The model under review builds one solid part; all positions refer to its coordinate system, in mm. A direction names the side the tool comes from. Give positions to 0.01 mm unless a question says otherwise; leave off trailing zeros. Loops run counter-clockwise (first coordinate to the right, second up) from the corner with the lowest first, then second, coordinate; pieces in that order, holes last. Notation, with made-up numbers: (73.5, -18.75) - (91.5, -18.75) arc R15 cw to (91.5, -0.75) - close; hole circle Ø6 at (32.5, 45). An arc over 180 degrees is marked (long way). Answer as a JSON object with one key per item and string values.
from build123d import *

# Parameters (mm, degrees)
SKETCH1_W           = 88
SKETCH1_H           = 18
BOSS_EXTRUDE1_DEPTH = 3.8
SKETCH2_W           = 18.8
SKETCH2_H           = 3.8
BOSS_EXTRUDE2_DEPTH = 3.8
SKETCH3_W           = 10
SKETCH3_H           = 3.8
BOSS_EXTRUDE3_DEPTH = 3.8
LPATTERN1_COUNT     = 3
LPATTERN1_PITCH     = 20
LPATTERN1_COL_COUNT = 3
LPATTERN1_COL_PITCH = 20
SKETCH4_W           = 1
SKETCH4_H           = 3.8
CUT_EXTRUDE1_DEPTH  = 92.709759568
SKETCH5_W           = 88
SKETCH5_H           = 3
BOSS_EXTRUDE4_DEPTH = 3.8
SKETCH6_W           = 5
SKETCH6_H           = 3.8
BOSS_EXTRUDE5_DEPTH = 3.8
SKETCH7_W           = 10
SKETCH7_H           = 7.6
BOSS_EXTRUDE6_DEPTH = 3.8
LPATTERN2_COUNT     = 3
LPATTERN2_PITCH     = 20
SKETCH9_W           = 9
SKETCH9_H           = 3.8
CUT_EXTRUDE2_DEPTH  = 92.506721065
SKETCH10_W          = 3.8
SKETCH10_H          = 5
SKETCH10_H_2        = 8
BOSS_EXTRUDE8_DEPTH = 3.8
SKETCH11_W          = 10
SKETCH11_H          = 3
CUT_EXTRUDE3_DEPTH  = 96.166800934


with BuildPart() as part:
    # Sketch1 → Boss-Extrude1 (new body)
    with BuildSketch(Plane(origin=(0, 0, 0), x_dir=(1, 0, 0), z_dir=(0, 1, 0))):
        with Locations((44, -9)):
            Rectangle(SKETCH1_W, SKETCH1_H)
    extrude(amount=BOSS_EXTRUDE1_DEPTH)

    # Sketch2 → Boss-Extrude2 (add, through all)
    with BuildSketch(Plane.XZ):
        with Locations((9.4, -1.9)):
            Rectangle(SKETCH2_W, SKETCH2_H)
    extrude(amount=-BOSS_EXTRUDE2_DEPTH)

    # Sketch3 → Boss-Extrude3 (add, through all)
    with BuildSketch(Plane.XZ):
        with Locations((44, 19.9)):
            Rectangle(SKETCH3_W, SKETCH3_H)
    boss_extrude3 = extrude(amount=-BOSS_EXTRUDE3_DEPTH)

    # LPattern1: Boss-Extrude3 ×3
    with Locations(*[(i * LPATTERN1_PITCH, 0, 0) for i in range(1, LPATTERN1_COUNT)]):
        add(boss_extrude3)

    # LPattern1 col: Boss-Extrude3 ×3
    with Locations(*[(-i * LPATTERN1_COL_PITCH, 0, 0) for i in range(1, LPATTERN1_COL_COUNT)]):
        add(boss_extrude3)

    # Sketch4 → Cut-Extrude1 (cut, through all)
    with BuildSketch(Plane(origin=(0, 0, 0), x_dir=(-1, 0, 0), z_dir=(0, -1, 0))):
        with Locations((0.5, -19.9)):
            Rectangle(SKETCH4_W, SKETCH4_H)
        with Locations((-88.5, -19.9)):
            Rectangle(SKETCH4_W, SKETCH4_H)
    extrude(amount=-CUT_EXTRUDE1_DEPTH, mode=Mode.SUBTRACT)

    # Sketch5 → Boss-Extrude4 (add, through all)
    with BuildSketch(Plane(origin=(0, 0, 0), x_dir=(-1, 0, 0), z_dir=(0, -1, 0))):
        with Locations((-44, -23.3)):
            Rectangle(SKETCH5_W, SKETCH5_H)
    extrude(amount=-BOSS_EXTRUDE4_DEPTH)

    # Sketch6 → Boss-Extrude5 (add, through all)
    with BuildSketch(Plane(origin=(0, 0, 0), x_dir=(-1, 0, 0), z_dir=(0, -1, 0))):
        with Locations((-2.5, 5.7)):
            Rectangle(SKETCH6_W, SKETCH6_H)
        with Locations((-16.3, 5.7)):
            Rectangle(SKETCH6_W, SKETCH6_H)
    extrude(amount=-BOSS_EXTRUDE5_DEPTH)

    # Sketch7 → Boss-Extrude6 (add, through all)
    with BuildSketch(Plane(origin=(0, 0, 0), x_dir=(-1, 0, 0), z_dir=(0, -1, 0))):
        with Locations((-83, 3.8)):
            Rectangle(SKETCH7_W, SKETCH7_H)
    boss_extrude6 = extrude(amount=-BOSS_EXTRUDE6_DEPTH)

    # LPattern2: Boss-Extrude6 ×3
    with Locations(*[(-i * LPATTERN2_PITCH, 0, 0) for i in range(1, LPATTERN2_COUNT)]):
        add(boss_extrude6)

    # Sketch9 → Cut-Extrude2 (cut, through all)
    with BuildSketch(Plane(origin=(0, 0, 0), x_dir=(-1, 0, 0), z_dir=(0, -1, 0))):
        with Locations((-4.5, -19.9)):
            Rectangle(SKETCH9_W, SKETCH9_H)
        with Locations((-83.5, -19.9)):
            Rectangle(SKETCH9_W, SKETCH9_H)
    extrude(amount=-CUT_EXTRUDE2_DEPTH, mode=Mode.SUBTRACT)

    # Sketch10 → Boss-Extrude8 (add, through all)
    with BuildSketch(Plane(origin=(0, 0, 0), x_dir=(-1, 0, 0), z_dir=(0, -1, 0))):
        with Locations((1.9, -11.7)):
            Rectangle(SKETCH10_W, SKETCH10_H)
        with Locations((-89.9, -9)):
            Rectangle(SKETCH10_W, SKETCH10_H_2)
        with Locations((1.9, -1.7)):
            Rectangle(SKETCH10_W, SKETCH10_H)
    extrude(amount=-BOSS_EXTRUDE8_DEPTH)

    # Sketch11 → Cut-Extrude3 (cut, through all)
    with BuildSketch(Plane(origin=(0, 0, 0), x_dir=(-1, 0, 0), z_dir=(0, -1, 0))):
        with Locations((-5, -23.3)):
            Rectangle(SKETCH11_W, SKETCH11_H)
        with Locations((-83, -23.3)):
            Rectangle(SKETCH11_W, SKETCH11_H)
    extrude(amount=-CUT_EXTRUDE3_DEPTH, mode=Mode.SUBTRACT)


solid = part.part
Q1. Consider section D-D, the plane y = 2.05. State how many separate pieces and enclosed holes the cut face has, plus the area to 3 significant figures.
Results:
{"separate pieces": "1", "enclosed holes": "2", "area": "2,310 mm^2"}
Q2. Clearance check with flat-ended pins moving along their axes: pin 1 Ø1.9 at (x, y) = (33.5, 3) entering from -Z; pin 2 Ø1.1 at (x, y) = (-2.5, 2.5) entering from -Z; pin 3 Ø1.1 at (y, z) = (1.5, 19.5) entering from +X. State where each tip first meets the part, or that it passes through.
Results:
{"pin 1": "stops at z = 0", "pin 2": "stops at z = -0.8", "pin 3": "stops at x = 69"}
Q3. Consider section C-C, the plane z = -5. State the section outline as (x, y) points.
Results:
{"outline": "(0, 0) - (5, 0) - (5, 3.8) - (0, 3.8) - close; (13.8, 0) - (18.8, 0) - (18.8, 3.8) - (13.8, 3.8) - close; (38, 0) - (48, 0) - (48, 3.8) - (38, 3.8) - close; (58, 0) - (68, 0) - (68, 3.8) - (58, 3.8) - close; (78, 0) - (88, 0) - (88, 3.8) - (78, 3.8) - close"}
Q4. The part is to be moulded in two halves that separate along Z. For faces 5 (the face through (-2, 2, 9.2)), 6 (the face through (13.8, 2, -6)), 7 (the face through (43, 2, -7.6)), say which applies: +Z half, -Z half, draft (parallel to the pull), parting line (faces both ways), or undercut.
Results:
{"face 5": "undercut", "face 6": "draft", "face 7": "-Z half"}
Q5. Consider section A-A, the plane x = 56.5. State the section outline as (y, z) points.
Results:
{"outline": "(0, 0) - (3.8, 0) - (3.8, 18) - (0, 18) - close; (0, 21.8) - (3.8, 21.8) - (3.8, 24.8) - (0, 24.8) - close"}
Q6. Consider section B-B, the plane z = 19.5. State the section outline as (x, y) points.
Results:
{"outline": "(19, 0) - (29, 0) - (29, 3.8) - (19, 3.8) - close; (39, 0) - (49, 0) - (49, 3.8) - (39, 3.8) - close; (59, 0) - (69, 0) - (69, 3.8) - (59, 3.8) - close"}
Q7. For faces 1 (the face through (90, 2, 5)), 2 (the face through (39, 2, 20)), 3 (the face through (0, 2, -4)), 4 (the face through (74, 2, 21.8)), list the 3-axis set-ups (+Z, -Z, +X, -X, +Y, -Y) from which the entire face can be reached by the end or side of a thin tool; tool diameter is ignored.
Results:
{"face 1": "-Z, +X, +Y, -Y", "face 2": "+Y, -Y", "face 3": "-Z, -X, +Y, -Y", "face 4": "+X, +Y, -Y"}
Q8. To check wall thickness, follow probe 1 along X at (y, z) = (0.35, 20.5); probe 2 along X at (y, z) = (1.85, -4); probe 3 along Z at (x, y) = (36, 0.3). State the ranges of each line that lie inside material, in increasing order. Write a range as [from, to].
Results:
{"probe 1": "x = [19, 29], [39, 49], [59, 69]", "probe 2": "x = [0, 5], [13.8, 18.8], [38, 48], [58, 68], [78, 88]", "probe 3": "z = [0, 18], [21.8, 24.8]"}
